Can you work these out from the model? Positions are in its coordinate system, mm. A direction names the side the tool comes from. Round coordinates to 2 decimals unless told otherwise and drop trailing zeros. Write each loop counter-clockwise with the first axis right and the second up, starting at its lowest first coordinate (ties: lowest second). Pieces come first, ordered by that corner, then holes. Notation, with made-up numbers: M -7.75,74 L 29.25,74 A4 ccw 29.25,81 Z; hole C 7,38.25 d9. An arc over 180 degrees is marked long. Answer in a Markdown table with one row per item. Add a question column.
(1) For faces 4 (the face through (-6.08, -0.91, 10.29)), 5 (the face through (-76.2, -6, 0)), 6 (the face through (-65, 0, 0)), 7 (the face through (33.452, -8, 0)), 8 (the face through (-47.625, 4, 0)), which set-ups out of +Z, -Z, +X, -X, +Y, -Y let a thin tool reach every point of the face, with its end or its side?
(2) If I drill on probe 1 along X at (y, z) = (-9.5, -2); probe 2 along X at (y, z) = (-7.5, -12); probe 3 along Y at (x, z) = (-6.5, 13), over which ranges is the centre line in solid material (lowest first)?
(3) Suppose I cut it at C-C, the plane x = -28. Write out the boundary of the cut face in (y, z), then the cut area to 3 significant figures.
(4) Suppose I cut it at B-B, the plane y = -4.75. Write out the boundary of the cut face in (x, z), then the cut area to 3 significant figures.
(5) Suppose I cut it at D-D, the plane y = 6. Write out the boundary of the cut face in (x, z) (3 decimals).
(6) If we mould it in two halves opening along Z, with no side actions, what happens to faces 1 (the face through (50.327, -0.905, 10.22)), 2 (the face through (-1, -6, 25.4)), 3 (the face through (-53.02, 10.21, 0.36))? For each: released by +Z, released by -Z, zero draft, split by the parting line, or undercut.
(7) Suppose I cut it at A-A, the plane z = -2. Count the separate pieces of the cut face and the enclosed holes in it, then the cut area to 3 significant figures.
(8) I'm going to push flat-ended pins straight in: pin 1 (6.5 mm diameter, centred on y = 5.5, z = -7.5, fed in from +X) (3 decimals); pin 2 (6.5 mm diameter, centred on y = 5.5, z = 1, fed in from -X) (3 decimals); pin 3 (24.5 mm diameter, centred on x = -64, z = -12.5, fed in from +Y). Where does each tip first touch, or does it pass through?
Autodesk Inventor part; units mm, degrees
ref_plane "YZ Plane" through (0, 0, 0) normal (1, 0, 0) x (0, 1, 0)
ref_plane "XZ Plane" through (0, 0, 0) normal (0, 1, 0) x (-1, 0, 0)
ref_plane "XY Plane" through (0, 0, 0) normal (0, 0, 1) x (1, 0, 0)
sketch "Sketch1" plane through (0, 0, 0) normal (0, 1, 0) x (-1, 0, 0)
  line L0 (-76.2, 25.4) -> (-76.2, -25.4)
  line L1 (-76.2, -25.4) -> (76.2, -25.4)
  line L2 (76.2, -25.4) -> (76.2, 25.4)
  line L3 (76.2, 25.4) -> (-76.2, 25.4)
  line L4 (-76.2, 25.4) -> (76.2, -25.4) construction
  line L5 (-76.2, -25.4) -> (76.2, 25.4) construction
  point P0 (0, 0)
  dimension "d0" = 50.8
  dimension "d1" = 152.4
extrude "Extrusion1" add sketch "Sketch1" against normal blind 12.7
sketch "Sketch2" plane through (0, 0, 0) normal (0, 1, 0) x (1, 0, 0)
  line L0 (-47.625, -25.4) -> (-47.625, 25.4)
  line L1 (-47.625, 25.4) -> (-53.975, 25.4)
  line L2 (-53.975, 25.4) -> (-53.975, -25.4)
  line L3 (-53.975, -25.4) -> (-47.625, -25.4)
  line L4 (-47.625, -25.4) -> (-53.975, 25.4) construction
  line L5 (-47.625, 25.4) -> (-53.975, -25.4) construction
  line L6 (-76.2, 25.4) -> (-76.2, -25.4)
  point P0 (0, 0)
  point P1 (-50.8, 0)
  dimension "d4" = 6.35
  dimension "d5" = 25.4
  dimension "d6" = 50.8
extrude "Extrusion2" add sketch "Sketch2" along normal blind 11.1125
fillet "Fillet1" radius 3.175 2 edges at (-47.625, 11.1125, 0) (-53.975, 11.1125, 0)
sketch "Sketch3" plane through (0, 0, 0) normal (0, 1, 0) x (1, 0, 0)
  line L0 (33.4515, -6.1606) -> (33.4515, 6.5394)
  line L1 (33.4515, 6.5394) -> (44.45, 12.8894)
  line L2 (44.45, 12.8894) -> (55.4485, 6.5394)
  line L3 (55.4485, 6.5394) -> (55.4485, -6.1606)
  line L4 (55.4485, -6.1606) -> (44.45, -12.5106)
  line L5 (44.45, -12.5106) -> (33.4515, -6.1606)
  line L6 (-10.9985, -6.35) -> (-10.9985, 6.35)
  line L7 (-10.9985, 6.35) -> (0, 12.7)
  line L8 (0, 12.7) -> (10.9985, 6.35)
  line L9 (10.9985, 6.35) -> (10.9985, -6.35)
  line L10 (10.9985, -6.35) -> (0, -12.7)
  line L11 (0, -12.7) -> (-10.9985, -6.35)
  line L12 (73.025, 22.225) -> (73.025, -22.225)
  point P0 (0, 0)
  point P1 (44.45, 0.1894)
  point P2 (0, 0)
  dimension "d12" = 25.4
  dimension "d13" = 44.45
extrude "Extrusion3" cut sketch "Sketch3" against normal through all
fillet "Fillet4" radius 3.175 12 edges at (49.9493, 0, 9.3356) (38.9507, 0, 9.3356) (33.4515, 0, -0.1894) (38.9507, 0, -9.7144) (49.9493, 0, -9.7144) (55.4485, 0, -0.1894) (10.9985, 0, 0) (5.4993, 0, 9.525) (-5.4993, 0, 9.525) (-10.9985, 0, 0) (-5.4993, 0, -9.525) (5.4993, 0, -9.525)
properties part number "Gap Guage"
Calculated:
| question | item | result |
|---|---|---|
| 1 | face 4 | +Y |
| 1 | face 5 | +Z, -Z, -X, +Y, -Y |
| 1 | face 6 | +Z, -Z, -X, +Y |
| 1 | face 7 | +Y, -Y |
| 1 | face 8 | +Z, -Z, +X, +Y |
| 2 | probe 1 | -76.2 to -11, 11 to 33.45, 55.45 to 76.2 |
| 2 | probe 2 | -76.2 to -1.21, 1.21 to 42.91, 45.99 to 76.2 |
| 2 | probe 3 | -12.7 to 0 |
| 3 | outline | M -12.7,-25.4 L 0,-25.4 L 0,25.4 L -12.7,25.4 Z |
| 3 | area | 645 mm² |
| 4 | outline | M -76.2,-25.4 L 76.2,-25.4 L 76.2,25.4 L -76.2,25.4 Z; hole M -11,-6.35 L 0,-12.7 L 11,-6.35 L 11,6.35 L 0,12.7 L -11,6.35 Z; hole M 33.45,-6.54 L 44.45,-12.89 L 55.45,-6.54 L 55.45,6.16 L 44.45,12.51 L 33.45,6.16 Z |
| 4 | area | 6,900 mm² |
| 5 | outline | M -53.975,-25.4 L -47.625,-25.4 L -47.625,25.4 L -53.975,25.4 Z |
| 6 | face 1 | undercut |
| 6 | face 2 | released by +Z |
| 6 | face 3 | zero draft |
| 7 | separate pieces | 3 |
| 7 | enclosed holes | 0 |
| 7 | area | 1,430 mm² |
| 8 | pin 1 | x = -47.625 |
| 8 | pin 2 | x = -53.975 |
| 8 | pin 3 | y = 10.97 |
